from build123d import *

# Parameters (mm, degrees)
SKETCH1_W           = 85
SKETCH1_H           = 35
BOSS_EXTRUDE1_DEPTH = 145.5
SKETCH4_R           = 12.75
CUT_EXTRUDE2_DEPTH  = 55
CUT_EXTRUDE3_DEPTH  = 156.705651792
SKETCH11_W          = 12
SKETCH11_H          = 25.5
CUT_EXTRUDE5_DEPTH  = 10
CUT_EXTRUDE6_DEPTH  = 2.5
SKETCH14_W          = 30
SKETCH14_H          = 10
SKETCH14_W_2        = 25
SKETCH14_H_2        = 5
BOSS_EXTRUDE2_DEPTH = 5
CUT_EXTRUDE12_REACH = 138.729
SKETCH16_W          = 85
SKETCH16_H          = 4.239608998


with BuildPart() as part:
    # Sketch1 → Boss-Extrude1 (new body)
    with BuildSketch(Plane(origin=(0, 0, 0), x_dir=(0, 0, -1), z_dir=(1, 0, 0))):
        with Locations((-0.5, 0)):
            Rectangle(SKETCH1_W, SKETCH1_H)
    extrude(amount=BOSS_EXTRUDE1_DEPTH)

    # Sketch4 → Cut-Extrude2 (cut)
    with BuildSketch(Plane.ZY):
        Circle(SKETCH4_R)
    extrude(amount=-CUT_EXTRUDE2_DEPTH, mode=Mode.SUBTRACT)

    # Sketch9 → Cut-Extrude3 (cut, through all)
    with BuildSketch(Plane(origin=(0, 17.5, 0), x_dir=(1, 0, 0), z_dir=(0, 1, 0))):
        Polygon((145.5, 42), (94, 42), (124.818014212, 16.5), (124.818014212, -17.5), (94, -43), (145.5, -43), align=None)
    extrude(amount=-CUT_EXTRUDE3_DEPTH, mode=Mode.SUBTRACT)

    # Sketch11 → Cut-Extrude5 (cut)
    with BuildSketch(Plane.XZ.offset(17.5)):
        with Locations((49, 0)):
            Rectangle(SKETCH11_W, SKETCH11_H)
    extrude(amount=-CUT_EXTRUDE5_DEPTH, mode=Mode.SUBTRACT)

    # Sketch12 → Cut-Extrude6 (cut)
    with BuildSketch(Plane.XZ.offset(17.5)):
        Polygon((50.974497594, 39.527447374), (48.784580707, 39.527447374), (18.473843114, 39.527447374), (18.473843114, 43), (14.973843114, 43), (14.973843114, 39.527447374), (14.973843114, 36.086149409), (47.474497594, 36.086149409), (47.474497594, 12.75), (50.974497594, 12.75), (50.974497594, 36.086149409), align=None)
    extrude(amount=-CUT_EXTRUDE6_DEPTH, mode=Mode.SUBTRACT)

    # Sketch14 → Boss-Extrude2 (add)
    # profile 1 of 2: a face of its own
    with BuildSketch(Plane.XZ.offset(17.5)):
        with Locations((47.067654603, -47)):
            Rectangle(SKETCH14_W, SKETCH14_H)
        with Locations((47.207687623, -47.202155092)):
            Rectangle(SKETCH14_W_2, SKETCH14_H_2, mode=Mode.SUBTRACT)
    # profile 2 of 2: a face of its own
    with BuildSketch(Plane.XZ.offset(17.5)):
        with Locations((47.067654603, 48)):
            Rectangle(SKETCH14_W, SKETCH14_H)
        with Locations((47.207687623, 48.202155092)):
            Rectangle(SKETCH14_W_2, SKETCH14_H_2, mode=Mode.SUBTRACT)
    extrude(amount=-BOSS_EXTRUDE2_DEPTH)

    # Sketch16 → Cut-Extrude12 (cut, up to next)
    with BuildSketch(Plane.ZY, mode=Mode.PRIVATE) as cut_extrude12_sk1:
        with Locations((0.5, 15.380195501)):
            Rectangle(SKETCH16_W, SKETCH16_H)
    cut_extrude12_tool1 = extrude(cut_extrude12_sk1.sketch, amount=-CUT_EXTRUDE12_REACH, mode=Mode.PRIVATE) & part.part
    add(cut_extrude12_tool1.solids().sort_by_distance((0, 15.380196, 0.5))[0], mode=Mode.SUBTRACT)


solid = part.part
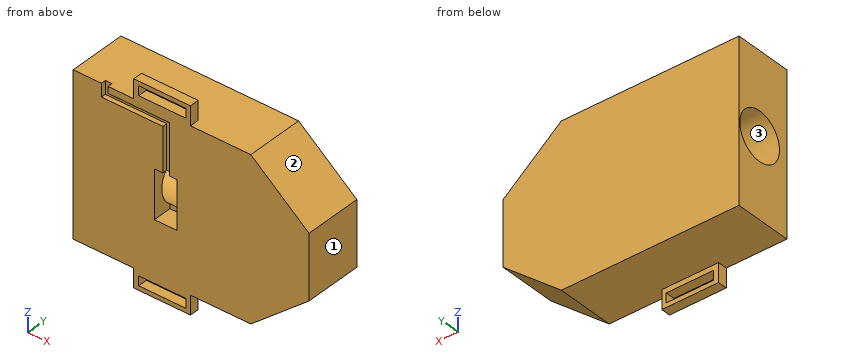
Input: part model. Units: mm. Frame: model coordinates. Face numbers are marked on the shaded views. Give positions to 0.01 mm unless a question says otherwise; leave off trailing zeros. Loops run counter-clockwise (first coordinate to the right, second up) from the corner with the lowest first, then second, coordinate; pieces in that order, holes last. Notation, with made-up numbers: (34.5, 86) -> (38.5, 86) arc R11 cw to (38.5, 100) -> close; hole circle Ø8 at (-4.5, 80.25). An arc over 180 degrees is marked (long way). Answer as a JSON object with one key per item and string values. Group by question number.
Item 1: Cut plane B-B, the plane x = 52.5. Return the cut outline in (y, z).
Item 2: Line query: probe 1 along Z at (x, y) = (40, 0); probe 2 along X at (y, z) = (-14.5, 6.5); probe 3 along Y at (x, z) = (15.5, 0). Output: solid intervals per line, ascending.
Item 3: Pull-direction query (Z, two-part tool) for the marked faces 1, 2 and 3; classes: released by +Z, released by -Z, zero draft, split by the parting line, or undercut.
Item 4: Pin query (flat end, axial travel): P1, Ø1.5, axis at y = -15.5, z = -47.5, coming from the +X side; P2, Ø6, axis at y = 10, z = 41, coming from the +X side; P3, Ø2.5, axis at y = -15.5, z = 49, coming from the -X side. Return the tip coordinate at first contact, or that it passes through.
Item 5: Cut plane C-C, the plane y = 0. Return the cut outline in (x, z), and give its area (3 significant figures).
Item 6: Cut plane D-D, the plane x = 69. Return the cut outline in (y, z), and give its area (3 significant figures).
Item 7: Cut plane A-A, the plane z = 0. Return the cut outline in (x, y), and give its area (3 significant figures).
Checks:
{
 "1": {"outline": "(-17.5, -52) -> (-12.5, -52) -> (-12.5, -49.7) -> (-17.5, -49.7) -> close; (-17.5, -44.7) -> (-12.5, -44.7) -> (-12.5, -42) -> (13.26, -42) -> (13.26, 43) -> (-12.5, 43) -> (-12.5, 45.7) -> (-17.5, 45.7) -> (-17.5, 12.75) -> (-7.5, 12.75) -> (-7.5, 10.31) arc R12.75 cw (long way) to (-7.5, -10.31) -> (-7.5, -12.75) -> (-17.5, -12.75) -> close; (-17.5, 50.7) -> (-12.5, 50.7) -> (-12.5, 53) -> (-17.5, 53) -> close"},
 "2": {"probe 1": "z = -42 to -12.75, 12.75 to 43", "probe 2": "x = 0 to 43, 55 to 124.82", "probe 3": "y = -17.5 to -12.75, 12.75 to 13.26"},
 "3": {"face 1": "zero draft", "face 2": "released by +Z", "face 3": "undercut"},
 "4": {"P1": "stops at x = 62.07", "P2": "stops at x = 100.04", "P3": "stops at x = 32.07"},
 "5": {"outline": "(0, -42) -> (94, -42) -> (124.82, -16.5) -> (124.82, 17.5) -> (94, 43) -> (0, 43) -> (0, 12.75) -> (55, 12.75) -> (55, -12.75) -> (0, -12.75) -> close", "area": "8,420 mm²"},
 "6": {"outline": "(-17.5, -42) -> (13.26, -42) -> (13.26, 43) -> (-17.5, 43) -> close", "area": "2,610 mm²"},
 "7": {"outline": "(0, -17.5) -> (43, -17.5) -> (43, -12.75) -> (0, -12.75) -> close; (0, 12.75) -> (55, 12.75) -> (55, -17.5) -> (124.82, -17.5) -> (124.82, 13.26) -> (0, 13.26) -> close", "area": "2,380 mm²"}
}
